Can you work these out from the model? Positions are in its coordinate system, mm. Give positions to 0.01 mm unless a question says otherwise; leave off trailing zeros. Write each loop counter-clockwise with the first axis right and the second up, starting at its lowest first coordinate (ties: lowest second). Pieces come first, ordered by that corner, then holes. Notation, with made-up numbers: (63, -27) - (104, -27) arc R21 cw to (104, -9) - close; hole circle Ø2 at (33.25, -0.75). An arc over 180 degrees is marked (long way). Return JSON: item names as keys, results as strings. Group by question number.
from build123d import *

# Parameters (mm, degrees)
F0_W     = 80
F0_H     = 100
F1_DEPTH = 100
F2_SIZE  = 20


with BuildPart() as f1:
    # F0 (on Top) → F1 (new body)
    with BuildSketch(Plane.XY):
        with Locations((40, -50)):
            Rectangle(F0_W, F0_H)
    extrude(amount=-F1_DEPTH)

    # F2
    f2_edges = [f1.edges().sort_by_distance(p)[0] for p in [
        (80, -50, -100),
        (40, -100, -100),
        (40, 0, -100),
        (0, -50, -100),
    ]]
    chamfer(f2_edges, length=F2_SIZE)


solid = f1.part
1) Will this pin go through, and if not, where does the flat tip stop? pin 1 Ø12 at (x, y) = (70.5, -79) entering from -Z.
2) Imagine slicing it at C-C, the plane z = -89. Write out the boundary of the cut face in (x, y).
3) Imagine slicing it at B-B, the plane x = 10. Write out the boundary of the cut face in (y, z), and give its area (3 significant figures).
4) Imagine slicing it at A-A, the plane y = -17. Write out the boundary of the cut face in (x, z), and give its area (3 significant figures).
5) I need wall thicknesses on line 1 along Z through (x, y) = (72.5, -83); line 2 along X through (y, z) = (-12, -83); line 3 along Z through (x, y) = (38.5, -13). Which ranges of each line are inside material? Lowest first, please.
Resolved:
{
 "1": {"pin 1": "z = -95.5"},
 "2": {"outline": "(9, -91) - (71, -91) - (71, -9) - (9, -9) - close"},
 "3": {"outline": "(-100, -80) - (-90, -90) - (-10, -90) - (0, -80) - (0, 0) - (-100, 0) - close", "area": "8,900 mm^2"},
 "4": {"outline": "(0, -80) - (17, -97) - (63, -97) - (80, -80) - (80, 0) - (0, 0) - close", "area": "7,470 mm^2"},
 "5": {"line 1": "-87.5 to 0", "line 2": "3 to 77", "line 3": "-93 to 0"}
}
